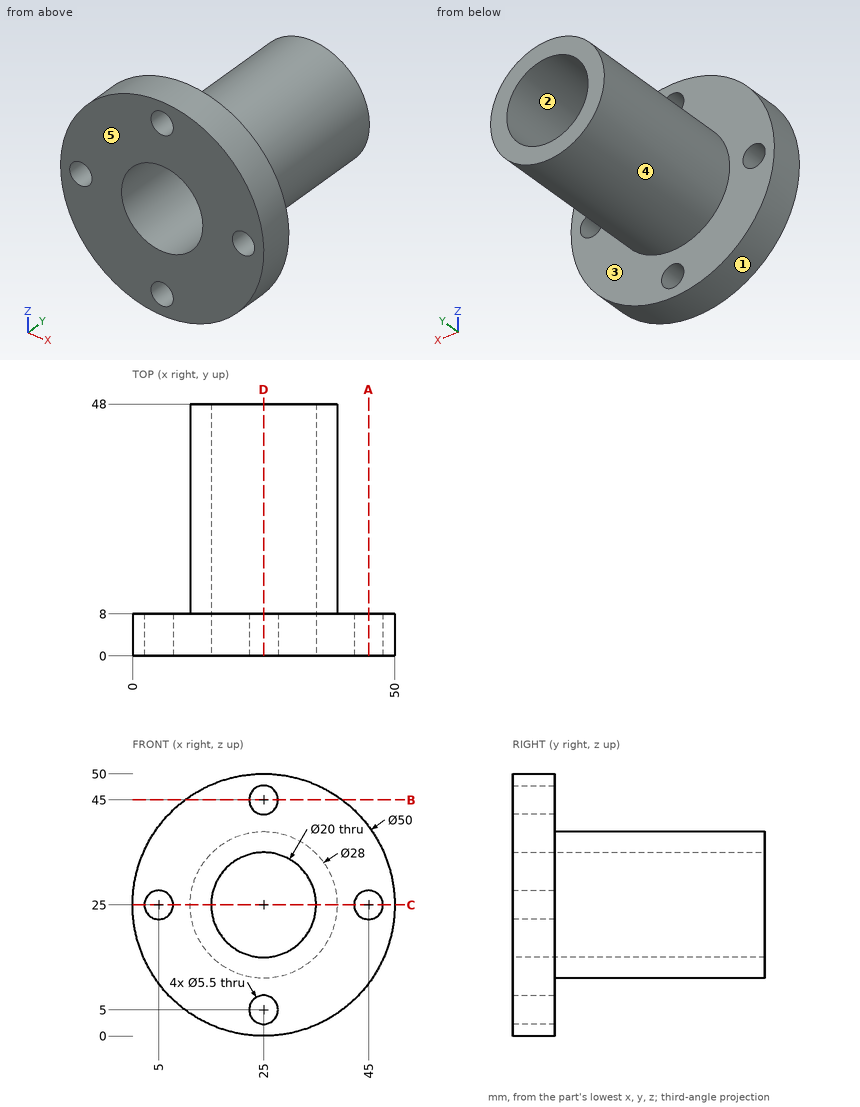
Here's the drawing with two shaded views (mm, measured from the low corner). I have some questions. A direction names the side the tool comes from. Give positions to 0.01 mm unless a question says otherwise; leave off trailing zeros. Loops run counter-clockwise (first coordinate to the right, second up) from the corner with the lowest first, then second, coordinate; pieces in that order, holes last. Notation, with made-up numbers: M 45,71 L 88,71 A20 ccw 88,106 Z; hole C 83.25,54 d3. An arc over 180 degrees is marked long. One line per item, written item: value. Start each with the question number.
1) I'm going to push flat-ended pins straight in: pin 1 (6 mm diameter, centred on x = 35.5, z = 43.5, fed in from +Y); pin 2 (8 mm diameter, centred on y = 5, z = 23.5, fed in from -X); pin 3 (6 mm diameter, centred on y = 13, z = 6, fed in from +X); pin 4 (12 mm diameter, centred on y = 13.5, z = 16.5, fed in from -X). Where does each tip first touch, or does it pass through?
2) If we section it at D-D, the plane x = 25: Write out the boundary of the cut face in (y, z).
3) If I drill on line 1 (X direction, y = 2, z = 25); line 2 (X direction, y = 19, z = 25); line 3 (Y direction, x = 5, z = 32), over which ranges is the centre line in solid material (lowest first)? Write a range as [from, to].
4) If we section it at A-A, the plane x = 45: Write out the boundary of the cut face in (y, z).
5) Thinking about a two-plate mould opening in Z: for the marked faces 1, 2 and 3, which applies, +Z half, -Z half, draft (parallel to the pull), parting line (faces both ways), or undercut?
6) On a 3-axis mill with a long thin cutter (end or side, diameter ignored), from which of +Z, -Z, +X, -X, +Y, -Y can I reach the whole of each face in a straight line? I mean the marked faces 4 and 5. Say none if no direction works.
7) If we section it at C-C, the plane z = 25: Write out the boundary of the cut face in (x, y), and give its area (3 significant figures).
8) If we section it at B-B, the plane z = 45: Write out the boundary of the cut face in (x, y).
Completed:
1. pin 1: stops at y = 8
1. pin 2: stops at x = 0
1. pin 3: passes through
1. pin 4: stops at x = 0.76
2. outline: M 0,0 L 8,0 L 8,2.25 L 0,2.25 Z; M 0,7.75 L 8,7.75 L 8,11 L 48,11 L 48,15 L 0,15 Z; M 0,35 L 48,35 L 48,39 L 8,39 L 8,42.25 L 0,42.25 Z; M 0,47.75 L 8,47.75 L 8,50 L 0,50 Z
3. line 1: x = [0, 2.25], [7.75, 15], [35, 42.25], [47.75, 50]
3. line 2: x = [11, 15], [35, 39]
3. line 3: y = [0, 8]
4. outline: M 0,10 L 8,10 L 8,22.25 L 0,22.25 Z; M 0,27.75 L 8,27.75 L 8,40 L 0,40 Z
5. face 1: parting line
5. face 2: undercut
5. face 3: draft
6. face 4: +Y
6. face 5: +Z, -Z, +X, -X, -Y
7. outline: M 0,0 L 2.25,0 L 2.25,8 L 0,8 Z; M 7.75,0 L 15,0 L 15,48 L 11,48 L 11,8 L 7.75,8 Z; M 35,0 L 42.25,0 L 42.25,8 L 39,8 L 39,48 L 35,48 Z; M 47.75,0 L 50,0 L 50,8 L 47.75,8 Z
7. area: 472 mm^2
8. outline: M 10,0 L 22.25,0 L 22.25,8 L 10,8 Z; M 27.75,0 L 40,0 L 40,8 L 27.75,8 Z
